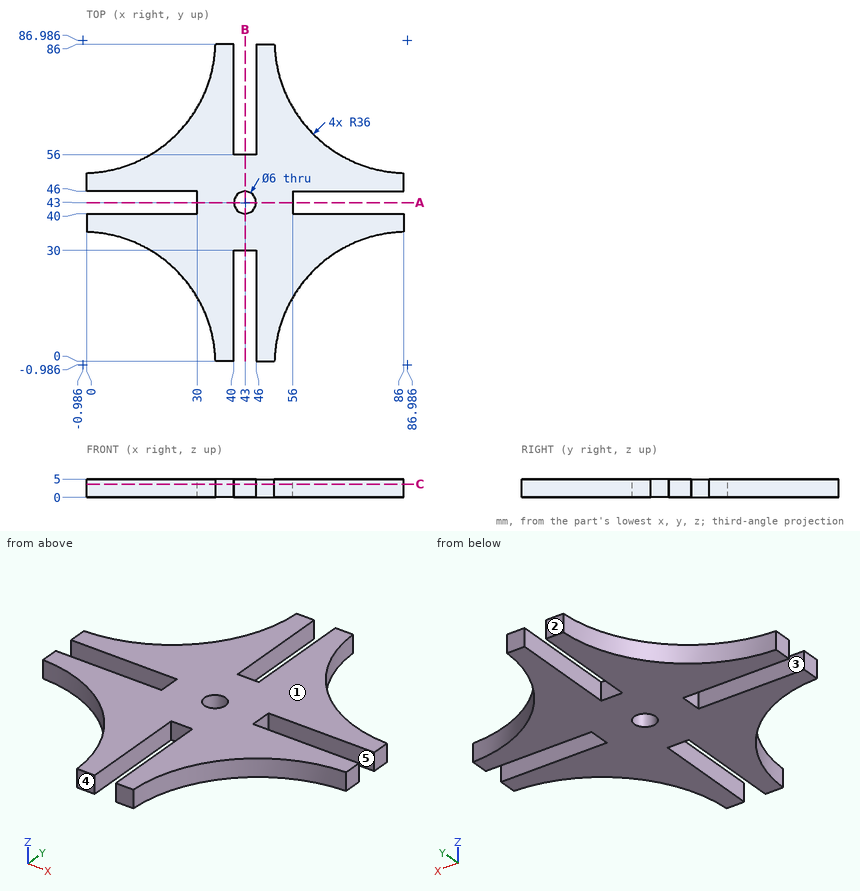
Input: dimensioned drawing with shaded views. Units: mm. Origin: part minimum x, y, z. A direction names the side the tool comes from. Coordinates: 2 decimals unless noted, no trailing zeros. Write each loop counter-clockwise with the first axis right and the second up, starting at its lowest first coordinate (ties: lowest second). Pieces come first, ordered by that corner, then holes. Notation, with made-up numbers: M 75,1 L 118,1 A21 cw 118,28 Z; hole C -37.75,23 d7. An arc over 180 degrees is marked long. Use one line per item in the form item = value.
Q1. Section C-C (z = 3.6). Return loops of the section in (x, y), plus the area to 3 significant figures.
Answer below:
outline = M 0,35 A36 cw 35,0 L 40,0 L 40,30 L 46,30 L 46,0 L 51,0 A36 cw 86,35 L 86,40 L 56,40 L 56,46 L 86,46 L 86,51 A36 cw 51,86 L 46,86 L 46,56 L 40,56 L 40,86 L 35,86 A36 cw 0,51 L 0,46 L 30,46 L 30,40 L 0,40 Z; hole C 43,43 d6
area = 2,860 mm²
Q2. First-contact query: pin 1 (2.5 mm diameter, centred on y = 42.5, z = 3, fed in from +X); pin 2 (2 mm diameter, centred on y = 17.5, z = 3.5, fed in from -X) (1 decimal); pin 3 (2.5 mm diameter, centred on x = 73.5, z = 1.5, fed in from -Y). Flat tips, straight axial feed; report the tip coordinate or a pass-through.
Answer below:
pin_1 = 56
pin_2 = 29.3
pin_3 = 31.86
Q3. Material intervals for probe 1 along Y at (x, z) = (43, 1.6); probe 2 along Y at (x, z) = (61.5, 3.2); probe 3 along X at (y, z) = (72.5, 4.6), sorted ascending. Write a range as from..to.
Answer below:
probe_1 = 30..40, 46..56
probe_2 = 24.44..40, 46..61.56
probe_3 = 31.97..40, 46..54.03
Q4. Section A-A (y = 43). Return loops of the section in (x, z), plus the area to 3 significant figures.
Answer below:
outline = M 30,0 L 40,0 L 40,5 L 30,5 Z; M 46,0 L 56,0 L 56,5 L 46,5 Z
area = 100 mm²
Q5. Draft query along Y for the marked faces 1, 2 and 3. Return one class per face: released by +Y, released by -Y, zero draft, split by the parting line, or undercut.
Answer below:
face_1 = zero draft
face_2 = released by +Y
face_3 = undercut
Q6. Set-up query: the marked faces 4 and 5. Return all of +Z, -Z, +X, -X, +Y, -Y with unobstructed straight access to the full face (end or side cutting, diameter ignored); none if empty.
Answer below:
face_4 = +Z, -Z, +X, -X, -Y
face_5 = +Z, -Z, +X
